For this review, use the dimensioned drawing (mm, ordinates from the lowest corner) and the shaded views. A direction names the side the tool comes from. Give positions to 0.01 mm unless a question says otherwise; leave off trailing zeros. Order: outer loops, then holes, each group sorted by start corner. A loop starts at its lowest first (then second) coordinate and runs counter-clockwise, first axis right, second up.
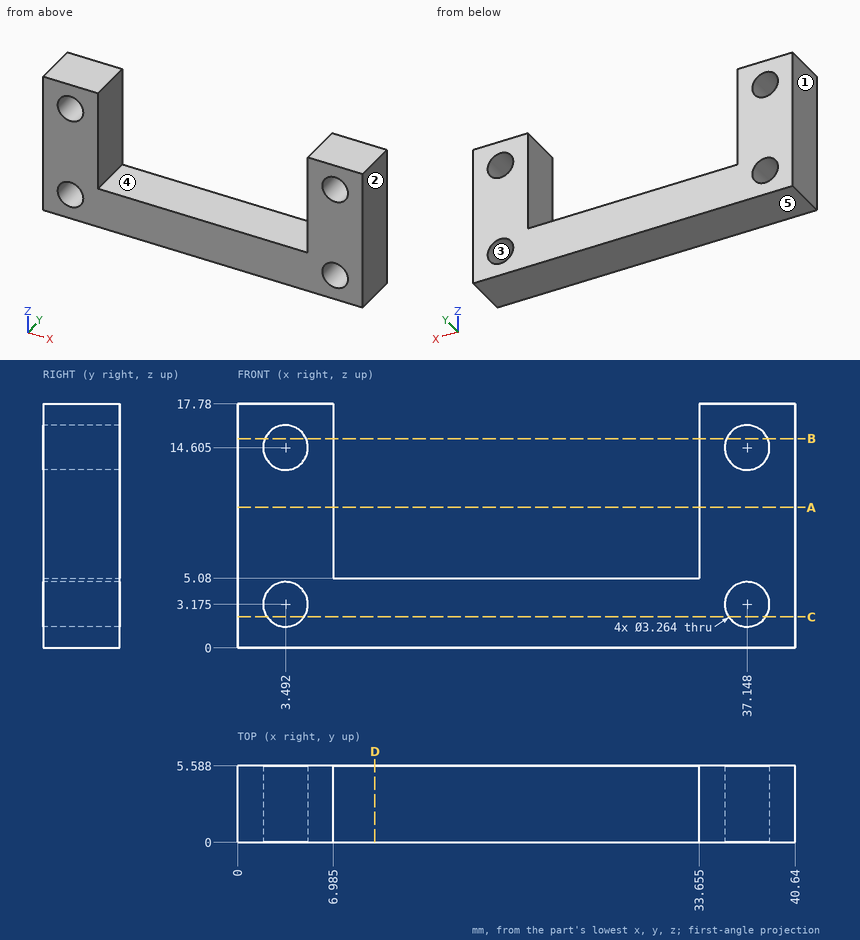
1. Take a section at C-C (z = 2.25). State the section outline as (x, y) points.
Recorded:
outline: (0, 0) - (2.15, 0) - (2.15, 5.59) - (0, 5.59) - close; (4.84, 0) - (35.8, 0) - (35.8, 5.59) - (4.84, 5.59) - close; (38.49, 0) - (40.64, 0) - (40.64, 5.59) - (38.49, 5.59) - close
2. Take a section at D-D (x = 10). State the section outline as (y, z) points, then the cut area to 3 significant figures.
Recorded:
outline: (0, 0) - (5.59, 0) - (5.59, 5.08) - (0, 5.08) - close
area: 28.4 mm2
3. Draft analysis for pull direction X (two halves, no side actions). For the marked faces 1, 2 and 3, state which applies: pulls with the +X half, pulls with the -X half, needs draft (parallel to the pull), parting line crosses it, or undercut.
Recorded:
face 1: pulls with the -X half
face 2: pulls with the +X half
face 3: undercut
4. For line 1 along X through (y, z) = (2.25, 16.5) (1 decimal); line 2 along Z through (x, y) = (3.5, 1.1); line 3 along X through (y, z) = (3.85, 15) (1 decimal), list the stretches that pass through material, from the lowest coordinate up.
Recorded:
line 1: x = 0 to 7, 33.7 to 40.6
line 2: z = 0 to 1.54, 4.81 to 12.97, 16.24 to 17.78
line 3: x = 0 to 1.9, 5.1 to 7, 33.7 to 35.6, 38.7 to 40.6
5. Take a section at B-B (z = 15.25). State the section outline as (x, y) points (1 decimal).
Recorded:
outline: (0, 0) - (2, 0) - (2, 5.6) - (0, 5.6) - close; (5, 0) - (7, 0) - (7, 5.6) - (5, 5.6) - close; (33.7, 0) - (35.6, 0) - (35.6, 5.6) - (33.7, 5.6) - close; (38.6, 0) - (40.6, 0) - (40.6, 5.6) - (38.6, 5.6) - close
6. Take a section at A-A (z = 10.25). State the section outline as (x, y) points (1 decimal).
Recorded:
outline: (0, 0) - (7, 0) - (7, 5.6) - (0, 5.6) - close; (33.7, 0) - (40.6, 0) - (40.6, 5.6) - (33.7, 5.6) - close
7. Machinability: for the marked faces 4 and 5, which of the approach directions +Z, -Z, +X, -X, +Y, -Y give a long, thin tool a straight path to every point of the face, cutting with its end or side? Answer none if there is none.
Recorded:
face 4: +Z, +Y, -Y
face 5: -Z, +X, -X, +Y, -Y
8. For pin 1 (3 mm diameter, centred on x = 7.5, y = 2, fed in from -Z); pin 2 (1.7 mm diameter, centred on x = 14.5, y = 3, fed in from +Z), all flat-tipped, find the tip position at first contact; note any pin that passes through.
Recorded:
pin 1: stops at z = 0
pin 2: stops at z = 5.08
